```python
from build123d import *

# Parameters (mm, degrees)
PAD005_DEPTH            = 4
SKETCH014_R             = 2.5
PAD006_DEPTH            = 2
CHAMFER_SIZE            = 0.25
BODY005_ROLL_ANGLE      = -51.0553562624
BODY005_PLACEMENT_ANGLE = 180


with BuildPart() as part:
    # Sketch013 → Pad005 (new body, symmetric)
    with BuildSketch(Plane.YZ):
        with BuildLine():
            ThreePointArc((0, 3), (-3, 0), (0, -3))
            Line((0, 3), (0, -3))
        make_face()
    extrude(amount=PAD005_DEPTH, both=True)

    # Sketch014 (on Face2 of Pad005) → Pad006 (join)
    with BuildSketch(Plane.ZX):
        Circle(SKETCH014_R)
    extrude(amount=PAD006_DEPTH)

    # Chamfer
    chamfer_edges = [part.edges().sort_by_distance(p)[0] for p in [
        (0, 2, -2.5),
        (-4, -3, 0),
        (-4, 0, 0),
        (4, -3, 0),
        (4, 0, 0),
        (0, 0, -3),
        (0, 0, 3),
    ]]
    chamfer(chamfer_edges, length=CHAMFER_SIZE)


with BuildPart() as part_1:
    # Body005 roll: moved
    add(part.part.rotate(Axis((0, 0, 0), (1, 0, 0)), BODY005_ROLL_ANGLE))


with BuildPart() as part_2:
    # Body005 placement: moved
    add(part_1.part.moved(Location((0, 23.5078988941, 19.0379414122))).rotate(Axis((0, 23.5078988941, 19.0379414122), (0, 0, 1)), BODY005_PLACEMENT_ANGLE))


solid = part_2.part
```
Verification items for the finished model (mm, model axes). Coordinates: 2 decimals unless noted, no trailing zeros. Loops run counter-clockwise (first coordinate to the right, second up) from the corner with the lowest first, then second, coordinate; pieces in that order, holes last. Notation, with made-up numbers: (88, -0.5) - (99, -0.5) arc R14 ccw to (99, 6.5) - close; hole circle Ø9 at (36, 36.5). An arc over 180 degrees is marked (long way). Put each result on its own line as item: value.
Item 1: Section check A-A (x = 3). Enter the section's corners in (y, z), then the cut area to 3 significant figures.
Conclusion:
outline: (21.34, 21.11) - (21.37, 20.77) - (25.65, 17.31) - (25.99, 17.35) arc R3 ccw to start
area: 14.1 mm2
Item 2: Draft check along Y on faces 1 (the face through (0.96, 21.17, 19.82)), 2 (the face through (-3.88, 23.56, 19.16)), 3 (the face through (-0.052, 25.345, 21.41)). Enter one of: pulls with the +Y half, pulls with the -Y half, needs draft (parallel to the pull), parting line crosses it, or undercut.
Conclusion:
face 1: undercut
face 2: pulls with the -Y half
face 3: parting line crosses it
Item 3: Scan lines: line 1 along Z through (x, y) = (-2, 25.75); line 2 along Y through (x, z) = (3.5, 19.65); line 3 along Z through (x, y) = (3, 25.5). Record each from-to range of solid material in increasing order.
Conclusion:
line 1: z = 17.32 to 21.03
line 2: y = 22.75 to 26.44
line 3: z = 17.43 to 21.28
Item 4: Gauge pin test, flat ends, axial feed: pin 1 Ø2 at (x, z) = (-3, 18.5) entering from -Y; pin 2 Ø3 at (x, z) = (0.5, 17) entering from +Y; pin 3 Ø1 at (x, z) = (1, 18.5) entering from -Y. Record the tip position at first contact, or that the pin passes through.
Conclusion:
pin 1: stops at y = 21.25
pin 2: stops at y = 26.46
pin 3: stops at y = 20.57
